Source: three-view drawing plus pictorial views. Frame: mm from the lowest corner of the part. A direction names the side the tool comes from. Coordinates: 2 decimals unless noted, no trailing zeros. Write each loop counter-clockwise with the first axis right and the second up, starting at its lowest first coordinate (ties: lowest second). Pieces come first, ordered by that corner, then holes. Notation, with made-up numbers: (51, -13) - (58, -13) arc R35 cw to (58, 26) - close; hole circle Ø8 at (39, 76). An arc over 180 degrees is marked (long way). Put each result on its own line as item: value.
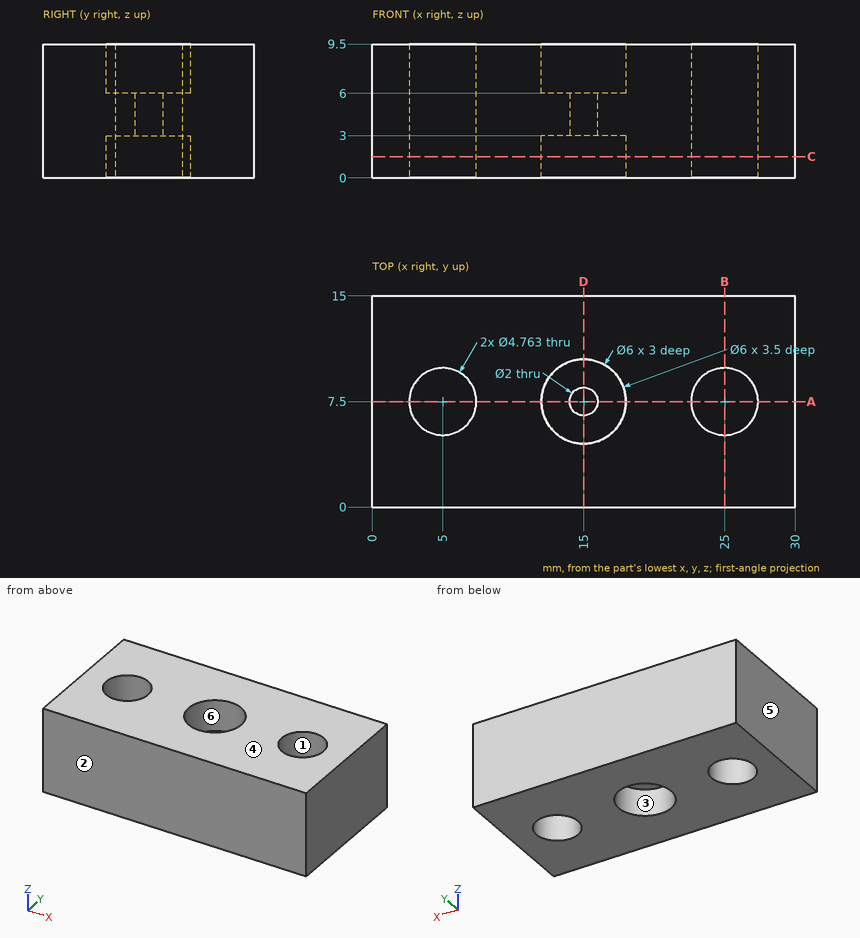
1. Section query D-D (x = 15). Return loops of the section in (y, z).
Answer below:
outline: (0, 0) - (4.5, 0) - (4.5, 3) - (6.5, 3) - (6.5, 6) - (4.5, 6) - (4.5, 9.5) - (0, 9.5) - close; (8.5, 3) - (10.5, 3) - (10.5, 0) - (15, 0) - (15, 9.5) - (10.5, 9.5) - (10.5, 6) - (8.5, 6) - close
2. Pin query (flat end, axial travel): pin 1 Ø3 at (x, y) = (5, 7.5) entering from +Z; pin 2 Ø7 at (x, y) = (15, 7.5) entering from -Z; pin 3 Ø1.8 at (x, y) = (15.5, 8) entering from +Z. Return the tip coordinate at first contact, or that it passes through.
Answer below:
pin 1: passes through
pin 2: stops at z = 0
pin 3: stops at z = 6
3. Section query A-A (y = 7.5). Return loops of the section in (x, z).
Answer below:
outline: (0, 0) - (2.62, 0) - (2.62, 9.5) - (0, 9.5) - close; (7.38, 0) - (12, 0) - (12, 3) - (14, 3) - (14, 6) - (12, 6) - (12, 9.5) - (7.38, 9.5) - close; (16, 3) - (18, 3) - (18, 0) - (22.62, 0) - (22.62, 9.5) - (18, 9.5) - (18, 6) - (16, 6) - close; (27.38, 0) - (30, 0) - (30, 9.5) - (27.38, 9.5) - close
4. Set-up query: the marked faces 5 and 6. Return all of +Z, -Z, +X, -X, +Y, -Y with unobstructed straight access to the full face (end or side cutting, diameter ignored); none if empty.
Answer below:
face 5: +Z, -Z, -X, +Y, -Y
face 6: +Z
5. Section query B-B (x = 25). Return loops of the section in (y, z).
Answer below:
outline: (0, 0) - (5.12, 0) - (5.12, 9.5) - (0, 9.5) - close; (9.88, 0) - (15, 0) - (15, 9.5) - (9.88, 9.5) - close
6. Section query C-C (z = 1.5). Return loops of the section in (x, y), then the cut area to 3 significant figures.
Answer below:
outline: (0, 0) - (30, 0) - (30, 15) - (0, 15) - close; hole circle Ø4.76 at (5, 7.5); hole circle Ø6 at (15, 7.5); hole circle Ø4.76 at (25, 7.5)
area: 386 mm²
7. Mould query, pull axis Y, two halves, no side actions, for the marked faces 1, 2, 3 and 4. Classes: +Y half, -Y half, draft (parallel to the pull), parting line (faces both ways), or undercut.
Answer below:
face 1: undercut
face 2: -Y half
face 3: undercut
face 4: draft
8. Ray query, probe 1 along X at (y, z) = (6.75, 2.25) (1 decimal); probe 2 along Y at (x, z) = (15, 1.05); probe 3 along X at (y, z) = (7.25, 5.5). Return the intervals inside material, ascending. Write a range as from..to.
Answer below:
probe 1: x = 0..2.7, 7.3..12.1, 17.9..22.7, 27.3..30
probe 2: y = 0..4.5, 10.5..15
probe 3: x = 0..2.63, 7.37..14.03, 15.97..22.63, 27.37..30
